For this review, take the finished solid that the model builds, in its own axes (mm). Face numbers are marked on the shaded views. A direction names the side the tool comes from. Coordinates: 2 decimals unless noted, no trailing zeros. Order: outer loops, then holes, each group sorted by start corner. A loop starts at its lowest first (then second) coordinate and runs counter-clockwise, first axis right, second up. Notation, with made-up numbers: (39, 0.25) -> (80, 0.25) arc R15 cw to (80, 17.25) -> close; hole circle Ø5 at (-23, 76.25). An arc over 180 degrees is marked (long way). Answer as a JSON object with one key per item and string values. Group by question number.
1) Add section D-D, the plane z = 28. Write out the cut boundary in (x, y).
2) For pin 1 (5 mm diameter, centred on x = -6, z = 54, fed in from +Y); pin 2 (3 mm diameter, centred on y = 0.5, z = 30, fed in from +X); pin 3 (5 mm diameter, centred on y = 2.5, z = 29, fed in from -X); pin 4 (4 mm diameter, centred on x = 1, y = -6, fed in from -Z), all flat-tipped, find the tip position at first contact; note any pin that passes through.
3) Machinability: for the marked faces 1 and 2, which of the approach directions +Z, -Z, +X, -X, +Y, -Y give a long, thin tool a straight path to every point of the face, cutting with its end or side? Answer none if there is none.
4) Wall thickness on L1, parallel to Z at x = -4.5, y = -5.5; L2, parallel to X at y = -3, z = 32; L3, parallel to Y at x = -2.25, z = 31: over which ranges is each line inside the solid? List them lowest first.
5) Add section C-C, the plane z = 54. Write out the cut boundary in (x, y).
6) Add section A-A, the plane x = 0. Write out the cut boundary in (y, z).
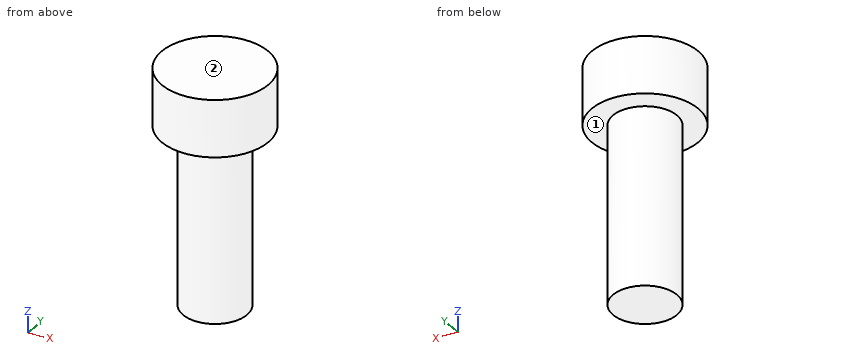
from build123d import *

# Parameters (mm, degrees)
CYLINDER014_R     = 4.5
CYLINDER014_DEPTH = 33
CYLINDER015_R     = 7.5
CYLINDER015_DEPTH = 8


with BuildPart() as cylinder014:
    # Cylinder014 → Cylinder014 (new body)
    with BuildSketch(Plane.XY.offset(25.5)):
        Circle(CYLINDER014_R)
    extrude(amount=CYLINDER014_DEPTH)


with BuildPart() as obj1:
    # Cylinder015 → Cylinder015 (new body)
    with BuildSketch(Plane.XY.offset(50.5)):
        Circle(CYLINDER015_R)
    extrude(amount=CYLINDER015_DEPTH)

    # Fusion004: union Cylinder014
    add(cylinder014.part)


solid = obj1.part
Output values:
{
 "1": {"outline": "circle Ø9 at (0, 0)"},
 "2": {"pin 1": "stops at y = 6.63", "pin 2": "stops at x = 4.5", "pin 3": "stops at x = -4.5", "pin 4": "stops at z = 25.5"},
 "3": {"face 1": "-Z", "face 2": "+Z, +X, -X, +Y, -Y"},
 "4": {"L1": "z = 50.5 to 58.5", "L2": "x = -3.35 to 3.35", "L3": "y = -3.9 to 3.9"},
 "5": {"outline": "circle Ø15 at (0, 0)"},
 "6": {"outline": "(-7.5, 50.5) -> (-4.5, 50.5) -> (-4.5, 25.5) -> (4.5, 25.5) -> (4.5, 50.5) -> (7.5, 50.5) -> (7.5, 58.5) -> (-7.5, 58.5) -> close"}
}
